Autodesk Inventor part; units mm, degrees
ref_plane "YZ Plane" through (0, 0, 0) normal (1, 0, 0) x (0, 1, 0)
ref_plane "XZ Plane" through (0, 0, 0) normal (0, 1, 0) x (-1, 0, 0)
ref_plane "XY Plane" through (0, 0, 0) normal (0, 0, 1) x (1, 0, 0)
sketch "Sketch1" plane through (0, 0, 0) normal (0, 1, 0) x (-1, 0, 0)
  circle A0 centre (0, 0) radius 8.5
  dimension "d0" = 17
extrude "Extrusion1" add sketch "Sketch1" along normal blind 3
sketch "Sketch2" plane through (0, 3, 0) normal (0, 1, 0) x (1, 0, 0)
  circle A0 centre (0, 0) radius 7.25
  dimension "d3" = 14.5
extrude "Extrusion2" add sketch "Sketch2" along normal blind 28
sketch "Sketch3" plane through (0, 31, 0) normal (0, 1, 0) x (1, 0, 0)
  circle A0 centre (0, 0) radius 6
  dimension "d6" = 12
extrude "Extrusion3" cut sketch "Sketch3" against normal blind 20
sketch "Sketch4" plane through (0, 0, 0) normal (0, -1, 0) x (1, 0, 0)
  circle A0 centre (0, 0) radius 3.5
  dimension "d10" = 7
extrude "Extrusion4" cut sketch "Sketch4" against normal blind 30.25
sketch "Sketch5" plane through (0, 31, 0) normal (0, 1, 0) x (1, 0, 0)
  point P0 (0, 0)
equation "\"BendRadius\" = Thickness"
equation "\"BendReliefWidth\" = Thickness"
equation "\"BendReliefDepth\" = 0.5 * Thickness"
equation "\"CornerReliefSize\" = 4 * Thickness"
equation "\"MinimumRemnant\" = 2 * Thickness"
equation "\"TransitionRadius\" = BendRadius"
equation "\"JacobiRadiusSize\" = BendRadius"
equation "\"GapSize\" = Thickness"
properties part number "Tornillo Caja 1"
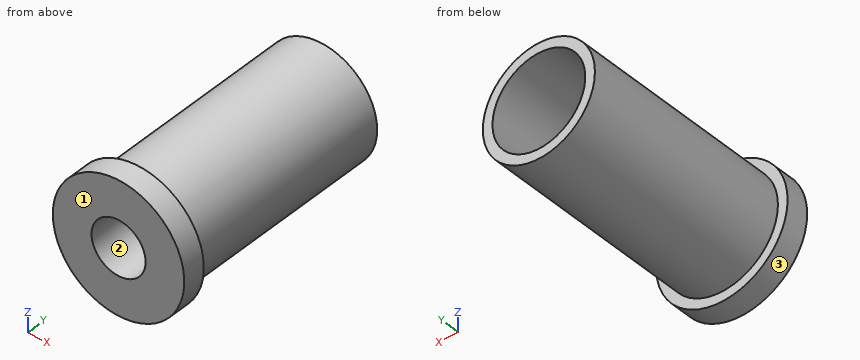
Geometry: final body of the model. Coordinates: model frame, mm. Face numbers are marked on the shaded views. Give positions to 0.01 mm unless a question says otherwise; leave off trailing zeros. Loops run counter-clockwise (first coordinate to the right, second up) from the corner with the lowest first, then second, coordinate; pieces in that order, holes last. Notation, with made-up numbers: (55, 35) -> (100, 35) arc R22 cw to (100, 59) -> close; hole circle Ø2 at (10.5, -28). An arc over 180 degrees is marked (long way). Use CSV: the item, a comma, the result in double quotes.
(1) Pull-direction query (X, two-part tool) for the marked faces 1, 2 and 3; classes: released by +X, released by -X, zero draft, split by the parting line, or undercut.
From the geometry:
face 1,"zero draft"
face 2,"undercut"
face 3,"split by the parting line"
(2) Cut plane B-B (z = 0). Output: boundary loops of the cut face in (x, y).
From the geometry:
outline,"(-8.5, 0) -> (-3.5, 0) -> (-3.5, 11) -> (-6, 11) -> (-6, 31) -> (-7.25, 31) -> (-7.25, 3) -> (-8.5, 3) -> close; (3.5, 0) -> (8.5, 0) -> (8.5, 3) -> (7.25, 3) -> (7.25, 31) -> (6, 31) -> (6, 11) -> (3.5, 11) -> close"
(3) Cut plane D-D (x = -4.5). Output: boundary loops of the cut face in (y, z).
From the geometry:
outline,"(0, -7.21) -> (3, -7.21) -> (3, -5.68) -> (31, -5.68) -> (31, -3.97) -> (11, -3.97) -> (11, 3.97) -> (31, 3.97) -> (31, 5.68) -> (3, 5.68) -> (3, 7.21) -> (0, 7.21) -> close"
(4) First-contact query: P1, Ø2, axis at x = -4, y = 20.5, coming from the +Z side; P2, Ø8, axis at x = 6, z = -2, coming from the -Y side; P3, Ø8.5, axis at x = -1, z = 0.5, coming from the +Y side; P4, Ø10, axis at x = -4, y = 26.5, coming from the -Z side. Flat tips, straight axial feed; report the tip coordinate or a pass-through.
From the geometry:
P1,"z = 6.6"
P2,"y = 0"
P3,"y = 11"
P4,"z = -7.25"
(5) Cut plane A-A (x = 0). Output: boundary loops of the cut face in (y, z).
From the geometry:
outline,"(0, -8.5) -> (3, -8.5) -> (3, -7.25) -> (31, -7.25) -> (31, -6) -> (11, -6) -> (11, -3.5) -> (0, -3.5) -> close; (0, 3.5) -> (11, 3.5) -> (11, 6) -> (31, 6) -> (31, 7.25) -> (3, 7.25) -> (3, 8.5) -> (0, 8.5) -> close"
(6) Cut plane C-C (y = 10). Output: boundary loops of the cut face in (x, z), plus the area to 3 significant figures.
From the geometry:
outline,"circle Ø14.5 at (0, 0); hole circle Ø7 at (0, 0)"
area,"127 mm^2"
(7) Ray query, line 1 along X through (y, z) = (25.5, 0); line 2 along Z through (x, y) = (0, 6.25). Return the intervals inside material, ascending. Write a range as [from, to].
From the geometry:
line 1,"[-7.25, -6], [6, 7.25]"
line 2,"[-7.25, -3.5], [3.5, 7.25]"
